```python
from build123d import *

# Parameters (mm, degrees)
SKETCH_1_R          = 1.5
EXTRUDE_1_DEPTH     = 2
SKETCH_2_R          = 2.625
EXTRUDE_2_DEPTH     = 2
FILLET_1_R          = 1
SKETCH_3_W          = 7.004697232
SKETCH_3_H          = 1
CUT_EXTRUDE_1_DEPTH = 1
SKETCH_4_W          = 1
SKETCH_4_H          = 3.75
CUT_EXTRUDE_2_DEPTH = 1


with BuildPart() as part:
    # Sketch 1 → Extrude 1 (new body)
    with BuildSketch(Plane(origin=(0, 0, 0), x_dir=(1, 0, 0), z_dir=(0, 1, 0))):
        with Locations(Location((0, 0, 0), (0, 0, 270))):
            Circle(SKETCH_1_R)
    extrude(amount=EXTRUDE_1_DEPTH)

    # Sketch 2 → Extrude 2 (add)
    with BuildSketch(Plane(origin=(0, 0, 0), x_dir=(-1, 0, 0), z_dir=(0, 1, 0))):
        with Locations(Location((0, 0, 0), (0, 0, 90))):
            Circle(SKETCH_2_R)
    extrude(amount=-EXTRUDE_2_DEPTH)

    # Fillet 1
    fillet_1_edges = [part.edges().sort_by_distance(p)[0] for p in [
        (0, -2, -2.625),
    ]]
    fillet(fillet_1_edges, radius=FILLET_1_R)

    # Sketch 3 → Cut-Extrude 1 (cut)
    with BuildSketch(Plane.XZ.offset(2)):
        Rectangle(SKETCH_3_W, SKETCH_3_H)
    extrude(amount=-CUT_EXTRUDE_1_DEPTH, mode=Mode.SUBTRACT)

    # Sketch 4 → Cut-Extrude 2 (cut)
    with BuildSketch(Plane.XZ.offset(2)):
        Rectangle(SKETCH_4_W, SKETCH_4_H)
    extrude(amount=-CUT_EXTRUDE_2_DEPTH, mode=Mode.SUBTRACT)


solid = part.part
```
The listing builds one solid part. Answer for the finished solid, in the listing's coordinates (mm). A direction names the side the tool comes from. Coordinates: 2 decimals unless noted, no trailing zeros. Loops run counter-clockwise (first coordinate to the right, second up) from the corner with the lowest first, then second, coordinate; pieces in that order, holes last. Notation, with made-up numbers: (87, 25.25) - (133, 25.25) arc R12 cw to (133, 42.25) - close; hole circle Ø4 at (-38.5, 41.25). An arc over 180 degrees is marked (long way). Use a Markdown table: item, result. Add a question column.
1) Given pin 1 (1.5 mm diameter, centred on x = 1.5, y = 0.5, fed in from -Z); pin 2 (0.5 mm diameter, centred on x = -1.5, y = -1.5, fed in from +Z); pin 3 (0.5 mm diameter, centred on x = 2, y = -1.5, fed in from +Z), each flat-ended and moving along its own axis, determine where each tip first touches the part or whether it passes through.
2) The part is cut by section C-C, the plane y = 0.15. Give the vertices of the cut face in (x, z), and give its area (3 significant figures).
3) The mould has two halves that part along X. Classify faces 1 (the flat face through (1, -2, 1)), 2 (the flat face through (0, -1, 0)), 3 (the cylindrical face through (0.45, 0.99, 1.43)): released by +X, released by -X, zero draft, split by the parting line, or undercut.
4) Find the intervals of material crossed by line 1 (X direction, y = -1.7, z = 1.4); line 2 (Y direction, x = 0.15, z = -1.55); line 3 (X direction, y = -0.5, z = -0.1), in increasing order.
5) For faces 4 (the flat face through (-1.6, -1.5, 0.5)), 5 (the flat face through (0, -1.5, 1.875)), 6 (the cylindrical face through (0.8, -0.5, 2.5)), 7 (the flat face through (1, -2, -1)), 8 (the flat face through (-2, 0, 0)), determine the directions among +Z, -Z, +X, -X, +Y, -Y from which every point of the face is accessible in a straight line to the end or side of a thin tool.
6) The part is cut by section B-B, the plane z = 0. Give the vertices of the cut face in (x, y) (3 decimals).
7) The part is cut by section A-A, the plane x = 0. Give the vertices of the cut face in (y, z) (3 decimals).
Here are the results:
| question | item | result |
|---|---|---|
| 1 | pin 1 | stops at z = -2.45 |
| 1 | pin 2 | stops at z = 2.21 |
| 1 | pin 3 | stops at z = 1.83 |
| 2 | outline | circle Ø3 at (0, 0) |
| 2 | area | 7.07 mm^2 |
| 3 | face 1 | zero draft |
| 3 | face 2 | undercut |
| 3 | face 3 | split by the parting line |
| 4 | line 1 | x = -1.87 to -0.5, 0.5 to 1.87 |
| 4 | line 2 | y = -1 to 0 |
| 4 | line 3 | x = -2.62 to 2.62 |
| 5 | face 4 | +X, -X, -Y |
| 5 | face 5 | -Y |
| 5 | face 6 | +Y, -Y |
| 5 | face 7 | +Z, -Z, +X, -X, -Y |
| 5 | face 8 | +Y |
| 6 | outline | (-2.625, -1) - (2.625, -1) - (2.625, 0) - (1.5, 0) - (1.5, 2) - (-1.5, 2) - (-1.5, 0) - (-2.625, 0) - close |
| 7 | outline | (-1.968, -1.875) arc R1 ccw to (-1, -2.625) - (0, -2.625) - (0, -1.5) - (2, -1.5) - (2, 1.5) - (0, 1.5) - (0, 2.625) - (-1, 2.625) arc R1 ccw to (-1.968, 1.875) - (-1, 1.875) - (-1, -1.875) - close |
